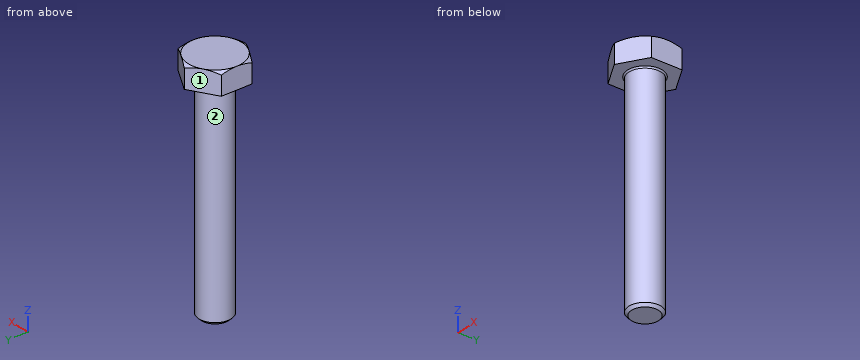
Autodesk Inventor part; units mm, degrees
ref_plane "WorkPlane1" through (0, 0, 0) normal (0, 0, 1) x (1, 0, 0)
ref_plane "MSC_PF1" through (0, 0, 0) normal (1, 0, 0) x (0, 1, 0)
ref_plane "MSC_PT1" through (0, 0, 0) normal (0, 0, -1) x (-1, 0, 0)
ref_plane "WorkPlane1" through (0, 0, 0) normal (0, 0, 1) x (1, 0, 0)
sketch "Szkic1" plane through (0, 0, 0) normal (0, 0, 1) x (1, 0, 0)
  point P0 (0, 0)
sketch "Szkic2" plane through (0, 0, 0) normal (0, 0, 1) x (1, 0, 0)
  line L0 (-5, 2.8868) -> (-5, -2.8868)
  line L1 (0, 5.7734) -> (-5, 2.8868)
  line L2 (5, 2.8868) -> (0, 5.7734)
  line L3 (5, -2.8868) -> (5, 2.8868)
  line L4 (0, -5.7734) -> (5, -2.8868)
  line L5 (-5, -2.8868) -> (0, -5.7734)
  circle A0 centre (0, 0) radius 5 construction
  dimension "d1" = 10
  dimension "d29" = 0
  dimension "d30" = 0
extrude "Wyciągnięcie proste1" add sketch "Szkic2" along normal blind 4
sketch "Szkic3" plane through (0, 0, 0) normal (1, 0, 0) x (0, 1, 0)
  line L0 (5, 4) -> (5.8734, 4)
  line L1 (5.8734, 3.4957) -> (5, 4)
  line L2 (5.8734, 4) -> (5.8734, 3.4957)
  line L3 (0, -0.8) -> (0, 4.8)
  line L4 (5.7734, 0) -> (5.7734, 4)
  dimension "d25" = 0.1
  dimension "d26" = 0
  dimension "d27" = 60
  dimension "d28" = 5
revolve "Obrót1" cut sketch "Szkic3" angle 360 about axis through (0, 0, -10) along (0, 0, 1)
sketch "Szkic4" plane through (0, 0, 0) normal (1, 0, 0) x (0, 1, 0)
  line L0 (0, -40) -> (0, 0)
  line L1 (-3, -40) -> (0, -40)
  line L2 (-3, 0) -> (-3, -40)
  line L3 (0, 0) -> (-3, 0)
  line L4 (0, -40) -> (0, 0)
  line L5 (-3.6, 0) -> (0.6, 0)
  line L6 (0, -48) -> (0, 8)
  dimension "d18" = 3
  dimension "d20" = 40
  dimension "d33" = 0
  dimension "d34" = 0
revolve "Obrót2" add sketch "Szkic4" angle 360 about axis through (0, 0, -40) along (0, 0, -1)
chamfer "Faza1" distance 0.5 angle 45 1 edges at (0, 3, -40)
fillet "Zaokrąglenie1" radius 0.25 1 edges at (0, 3, 0)
thread "Gwint1"
ref_plane "MSC_PF1" through (0, 0, 0) normal (1, 0, 0) x (0, 1, 0)
ref_plane "MSC_PT1" through (0, 0, 0) normal (0, 0, -1) x (-1, 0, 0)
equation "\"d1\" = ParS"
equation "\"d6\" = ParK"
equation "\"d22\" = 0.5 * PTC"
equation "\"d23\" = 0.5 * PTC"
equation "\"d24\" = r"
equation "\"d28\" = 0.5 * ParS"
equation "\"d18\" = 0.5 * NND"
equation "\"d20\" = NLG"
equation "\"NND\" = 6"
equation "\"NLG\" = 40"
equation "\"PTC\" = 1"
equation "\"ParK\" = 4"
equation "\"ParS\" = 10"
equation "\"msp_es\" = 0.577367 * ParS"
equation "\"r\" = 0.25"
equation "\"THREADDIA\" = NND"
properties part number "ISO 4016 - M6 x 40" material "Stal"
The model under review builds one solid part; all positions refer to its coordinate system, in mm. Face numbers are marked on the shaded views. A direction names the side the tool comes from. Round coordinates to 2 decimals unless told otherwise and drop trailing zeros. Write each loop counter-clockwise with the first axis right and the second up, starting at its lowest first coordinate (ties: lowest second). Pieces come first, ordered by that corner, then holes. Notation, with made-up numbers: M 50.25,55.5 L 95.25,55.5 A16 cw 95.25,80.5 Z; hole C 76.25,79 d11. An arc over 180 degrees is marked long. Use a Markdown table: item, result. Add a question column.
Q1. To check wall thickness, follow line 1 (Z direction, x = 0.25, y = 3.75); line 2 (Z direction, x = 0.75, y = -2.5); line 3 (Y direction, x = 2, z = -11). State the ranges of each line that lie inside material, in increasing order.
Q2. Machinability: for the marked faces 1 and 2, which of the approach directions +Z, -Z, +X, -X, +Y, -Y give a long, thin tool a straight path to every point of the face, cutting with its end or side? Answer none if there is none.
Q3. Insertion check: pin 1 (2 mm diameter, centred on y = -3, z = -26, fed in from -X); pin 2 (5 mm diameter, centred on x = -2, z = -31.5, fed in from +Y); pin 3 (6 mm diameter, centred on y = 3.5, z = -8.5, fed in from -X). Each pin has a flat end and moves straight along its axis. Give the tip position at first contact, or say it passes through.
Q4. We need section A-A, the plane z = -27. State the section outline as (x, y) points.
Findings below:
| question | item | result |
|---|---|---|
| 1 | line 1 | z = 0 to 4 |
| 1 | line 2 | z = -39.89 to 4 |
| 1 | line 3 | y = -2.24 to 2.24 |
| 2 | face 1 | +Z, -Z, -X, +Y |
| 2 | face 2 | -Z |
| 3 | pin 1 | stops at x = -2.24 |
| 3 | pin 2 | stops at y = 3 |
| 3 | pin 3 | stops at x = -2.96 |
| 4 | outline | C 0,0 d6 |
